Here's the drawing with two shaded views (mm, measured from the low corner). I have some questions. A direction names the side the tool comes from. Coordinates: 2 decimals unless noted, no trailing zeros. Loops run counter-clockwise (first coordinate to the right, second up) from the corner with the lowest first, then second, coordinate; pieces in that order, holes last. Notation, with made-up numbers: (9.5, -29) - (59.5, -29) arc R20 cw to (59.5, -16) - close; hole circle Ø7 at (17, -13.75). An arc over 180 degrees is marked (long way). One line per item, written item: value. Start each with the question number.
(1) On a 3-axis mill with a long thin cutter (end or side, diameter ignored), from which of +Z, -Z, +X, -X, +Y, -Y can I reach the whole of each face in a straight line? I mean the marked faces 1 and 2. Say none if no direction works.
(2) If we section it at A-A on x = 6.5: Write out the boundary of the cut face in (y, z), then the cut area to 3 significant figures.
(3) If I drill on line 1 along Y through (x, z) = (6.5, 40); line 2 along Z through (x, y) = (7.25, 8); line 3 along Z through (x, y) = (6.5, 5.25), over which ranges is the centre line in solid material (lowest first)? Write a range as from..to.
(4) If we section it at C-C on y = 2.25: Write out the boundary of the cut face in (x, z).
(5) If we section it at B-B on z = 20: Write out the boundary of the cut face in (x, y).
(6) I'm going to push flat-ended pins straight in: P1, Ø6, axis at x = 2, z = 15, coming from the -Y side; P2, Ø4, axis at y = 2, z = 19.5, coming from the +X side; P3, Ø1, axis at y = 2, z = 37.5, coming from the -X side. Where does each tip first touch, or does it pass through?
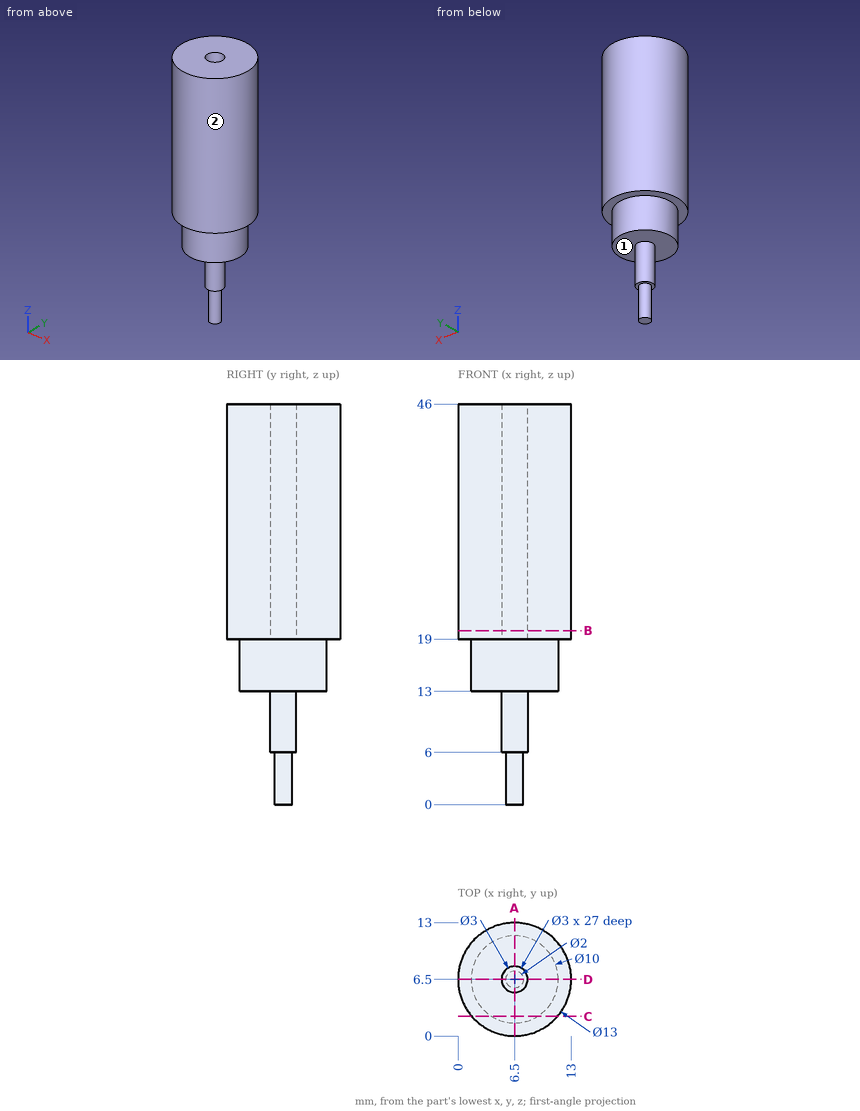
Values:
1. face 1: -Z
1. face 2: +Z, -Z
2. outline: (0, 19) - (1.5, 19) - (1.5, 13) - (5, 13) - (5, 6) - (5.5, 6) - (5.5, 0) - (7.5, 0) - (7.5, 6) - (8, 6) - (8, 13) - (11.5, 13) - (11.5, 19) - (13, 19) - (13, 46) - (8, 46) - (8, 19) - (5, 19) - (5, 46) - (0, 46) - close
2. area: 363 mm2
3. line 1: y = 0..5, 8..13
3. line 2: z = 13..46
3. line 3: z = 6..19
4. outline: (1.58, 19) - (3.87, 19) - (3.87, 13) - (9.13, 13) - (9.13, 19) - (11.42, 19) - (11.42, 46) - (1.58, 46) - close
5. outline: circle Ø13 at (6.5, 6.5); hole circle Ø3 at (6.5, 6.5)
6. P1: stops at y = 1.73
6. P2: stops at x = 12.5
6. P3: stops at x = 1.38
